Part model, mm, in its own coordinate system. Face numbers are marked on the shaded views. A direction names the side the tool comes from. Round coordinates to 2 decimals unless told otherwise and drop trailing zeros. Loops run counter-clockwise (first coordinate to the right, second up) from the corner with the lowest first, then second, coordinate; pieces in that order, holes last. Notation, with made-up numbers: (-22, 19.5) -> (14, 19.5) arc R12 ccw to (14, 27.5) -> close; hole circle Ø10 at (-37, 27). An arc over 180 degrees is marked (long way). Use a Markdown table: item, result. Add a question column.
Item 1: Which spindle directions (+Z, -Z, +X, -X, +Y, -Y) get a long thin tool onto all of the face, cutting with end or side? Do the marked faces 1 and 2. Say none if no direction does.
Item 2: Probe line 1 (Y direction, x = 0.25, z = 6); line 2 (Y direction, x = 3, z = 0.5); line 3 (Z direction, x = -8, y = 19.5). List the from-to ranges inside material, lowest first. Write a range as [from, to].
Item 3: Cut at D-D, the plane y = 36. List the corners of the cut face in (x, z).
Item 4: Cut at B-B, the plane z = 0. List the corners of the cut face in (x, y), plus the area to 4 significant figures.
Item 5: Cut at C-C, the plane y = 21.5. List the corners of the cut face in (x, z).
Item 6: Cut at A-A, the plane x = 0. List the corners of the cut face in (y, z).
Item 7: Flat gauge pins, fed straight in: pin 1 (10 mm diameter, centred on x = 7, y = 12.5, fed in from +Z); pin 2 (3 mm diameter, centred on y = 23, z = 0, fed in from +X); pin 3 (4 mm diameter, centred on x = 2.5, y = 31, fed in from +Z). Where does each tip first touch, or does it go through?
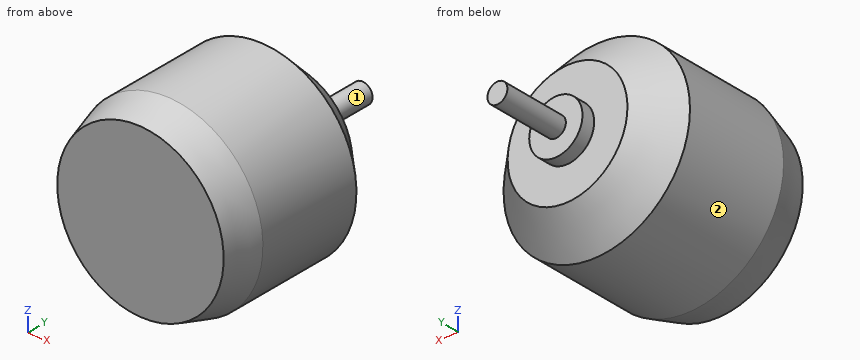
Autodesk Inventor part; units mm, degrees
ref_plane "YZ Plane" through (0, 0, 0) normal (1, 0, 0) x (0, 1, 0)
ref_plane "XZ Plane" through (0, 0, 0) normal (0, 1, 0) x (-1, 0, 0)
ref_plane "XY Plane" through (0, 0, 0) normal (0, 0, 1) x (1, 0, 0)
sketch "Boceto1" plane through (0, 0, 0) normal (0, 1, 0) x (-1, 0, 0)
  circle A0 centre (0, 0) radius 14
  dimension "d0" = 28
extrude "Extrusión1" add sketch "Boceto1" along normal blind 26
sketch "Boceto2" plane through (0, 26, 0) normal (0, 1, 0) x (1, 0, 0)
  circle A0 centre (0, 0) radius 4
  dimension "d3" = 8
extrude "Extrusión2" add sketch "Boceto2" along normal blind 2
sketch "Boceto3" plane through (0, 28, 0) normal (0, 1, 0) x (1, 0, 0)
  circle A0 centre (0, 0) radius 1.5
  dimension "d6" = 3
extrude "Extrusión3" add sketch "Boceto3" along normal blind 10
sketch "Boceto4" plane through (0, 0, 0) normal (1, 0, 0) x (0, 1, 0)
  line L0 (26, -14) -> (26, 14)
  line L1 (26, 14) -> (26, 9)
  line L2 (0, 14) -> (26, 14)
  line L3 (21, 14) -> (26, 9)
  line L4 (26, 14) -> (21, 14)
  line L5 (29.3126, 0) -> (24.3126, 0)
  line L6 (0, -14) -> (0, 14)
  line L7 (0, 14) -> (0, 12.5)
  line L8 (0, 14) -> (5, 14)
  line L9 (0, 14) -> (26, 14)
  line L10 (5, 14) -> (0, 12.5)
  point P0 (0, 0)
  dimension "d9" = 5
  dimension "d11" = 5
  dimension "d13" = 1.5
  dimension "d14" = 5
revolve "Revolución1" cut sketch "Boceto4" angle 360 about axis through (0, 29.3126, 0) along (0, -1, 0)
properties part number "Motor"
A:
| question | item | result |
|---|---|---|
| 1 | face 1 | +Y |
| 1 | face 2 | +Y, -Y |
| 2 | line 1 | y = [0, 26] |
| 2 | line 2 | y = [0, 28] |
| 2 | line 3 | z = [-11.49, 11.49] |
| 3 | outline | circle Ø3 at (0, 0) |
| 4 | outline | (-14, 5) -> (-12.5, 0) -> (12.5, 0) -> (14, 5) -> (14, 21) -> (9, 26) -> (4, 26) -> (4, 28) -> (1.5, 28) -> (1.5, 38) -> (-1.5, 38) -> (-1.5, 28) -> (-4, 28) -> (-4, 26) -> (-9, 26) -> (-14, 21) -> close |
| 4 | area | 741.5 mm^2 |
| 5 | outline | circle Ø27 at (0, 0) |
| 6 | outline | (0, -12.5) -> (5, -14) -> (21, -14) -> (26, -9) -> (26, -4) -> (28, -4) -> (28, -1.5) -> (38, -1.5) -> (38, 1.5) -> (28, 1.5) -> (28, 4) -> (26, 4) -> (26, 9) -> (21, 14) -> (5, 14) -> (0, 12.5) -> close |
| 7 | pin 1 | stops at z = 13.86 |
| 7 | pin 2 | stops at x = 13.5 |
| 7 | pin 3 | stops at z = 1.41 |
